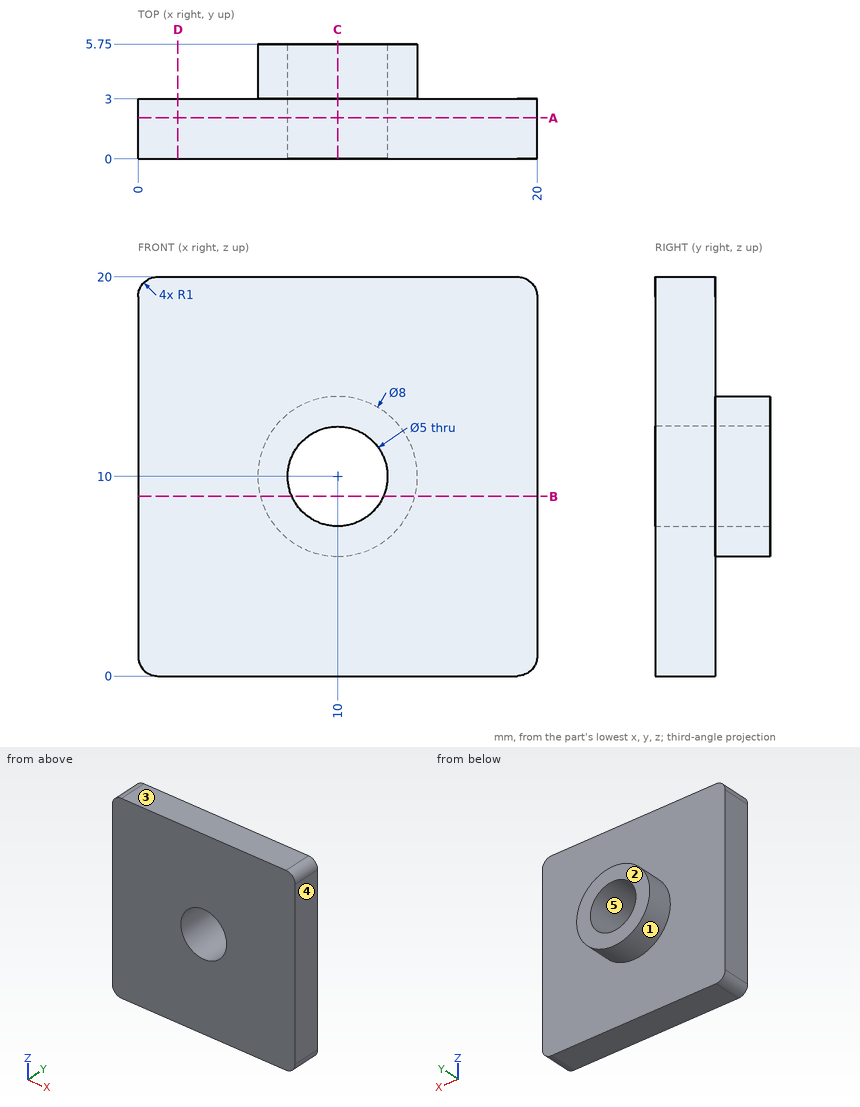
Study the drawing (mm; zero at the part's minimum x, y, z) and answer. A direction names the side the tool comes from. Give positions to 0.01 mm unless a question says otherwise; leave off trailing zeros. Write each loop counter-clockwise with the first axis right and the second up, starting at its lowest first coordinate (ties: lowest second). Pieces come first, ordered by that corner, then holes. Notation, with made-up numbers: (44.5, 44) -> (65.5, 44) arc R22 ccw to (65.5, 70) -> close; hole circle Ø2 at (61.25, -24.5). An arc over 180 degrees is marked (long way). Answer as a JSON object with one key per item and string values. Group by question number.
1) Find section B-B (z = 9). Write down the section's boundary in (x, y), and give its area (3 significant figures).
2) A tool of negligible diameter and unlimited length cuts with its end or side. For the marked faces 1 and 2, from which of +Z, -Z, +X, -X, +Y, -Y can it reach the whole face along a straight path? Write none if from no direction.
3) Find section D-D (x = 2). Write down the section's boundary in (y, z).
4) Find section A-A (y = 2.05). Write down the section's boundary in (x, z), and give its area (3 significant figures).
5) Consider L1, parallel to X at y = 3.8, z = 10; L2, parallel to X at y = 1.55, z = 10; L3, parallel to Y at x = 4.5, z = 12. Determine where each line is inside the solid, lowest interval first. Write a range as from..to.
6) Find section C-C (x = 10). Write down the section's boundary in (y, z), and give its area (4 significant figures).
7) Each of these flat-tipped pins is pushed along its axis until it touches: P1, Ø12, axis at x = 15, z = 17, coming from the +Y side; P2, Ø4.5, axis at x = 10, z = 10, coming from the +Y side. Where does it stop, or does it pass through?
8) The mould has two halves that part along Z. Classify the marked faces 3, 4 and 5: +Z half, -Z half, draft (parallel to the pull), parting line (faces both ways), or undercut.
Values follow:
{
 "1": {"outline": "(0, 0) -> (7.71, 0) -> (7.71, 5.75) -> (6.13, 5.75) -> (6.13, 3) -> (0, 3) -> close; (12.29, 0) -> (20, 0) -> (20, 3) -> (13.87, 3) -> (13.87, 5.75) -> (12.29, 5.75) -> close", "area": "55.0 mm2"},
 "2": {"face 1": "+Y", "face 2": "+Z, -Z, +X, -X, +Y"},
 "3": {"outline": "(0, 0) -> (3, 0) -> (3, 20) -> (0, 20) -> close"},
 "4": {"outline": "(0, 1) arc R1 ccw to (1, 0) -> (19, 0) arc R1 ccw to (20, 1) -> (20, 19) arc R1 ccw to (19, 20) -> (1, 20) arc R1 ccw to (0, 19) -> close; hole circle Ø5 at (10, 10)", "area": "380 mm2"},
 "5": {"L1": "x = 6..7.5, 12.5..14", "L2": "x = 0..7.5, 12.5..20", "L3": "y = 0..3"},
 "6": {"outline": "(0, 0) -> (3, 0) -> (3, 6) -> (5.75, 6) -> (5.75, 7.5) -> (0, 7.5) -> close; (0, 12.5) -> (5.75, 12.5) -> (5.75, 14) -> (3, 14) -> (3, 20) -> (0, 20) -> close", "area": "53.25 mm2"},
 "7": {"P1": "stops at y = 5.75", "P2": "passes through"},
 "8": {"face 3": "+Z half", "face 4": "draft", "face 5": "undercut"}
}
